Part model, mm, in its own coordinate system. A direction names the side the tool comes from. Give positions to 0.01 mm unless a question says otherwise; leave off trailing zeros. Loops run counter-clockwise (first coordinate to the right, second up) from the corner with the lowest first, then second, coordinate; pieces in that order, holes last. Notation, with made-up numbers: (26.25, -16) -> (31.25, -16) arc R25 cw to (31.25, -2) -> close; hole circle Ø9 at (8.25, 69). An arc over 180 degrees is marked (long way). Write item = value, one per line.
from build123d import *

# Parameters (mm, degrees)
BOSS_EXTRUDE1_DEPTH = 3
SKETCH2_R           = 16
BOSS_EXTRUDE2_DEPTH = 32
SKETCH3_R           = 13.8
BOSS_EXTRUDE3_DEPTH = 38
SKETCH4_R           = 18
SKETCH4_R_2         = 13.8
BOSS_EXTRUDE4_DEPTH = 17


with BuildPart() as part:
    # Sketch1 → Boss-Extrude1 (new body)
    with BuildSketch(Plane.XY):
        with BuildLine():
            Line((-4.002811512, 9), (4.002811512, 9))
            ThreePointArc((4.002811512, 9), (9.85, 0), (4.002811512, -9))
            Line((4.002811512, -9), (-4.002811512, -9))
            ThreePointArc((-4.002811512, -9), (-9.85, 0), (-4.002811512, 9))
        make_face()
    extrude(amount=BOSS_EXTRUDE1_DEPTH)

    # Sketch2 → Boss-Extrude2 (add)
    with BuildSketch(Plane(origin=(0, 0, 0), x_dir=(-1, 0, 0), z_dir=(0, 0, -1))):
        Circle(SKETCH2_R)
    extrude(amount=BOSS_EXTRUDE2_DEPTH)

    # Sketch3 → Boss-Extrude3 (add)
    with BuildSketch(Plane(origin=(0, 0, -32), x_dir=(-1, 0, 0), z_dir=(0, 0, -1))):
        Circle(SKETCH3_R)
    extrude(amount=BOSS_EXTRUDE3_DEPTH)

    # Sketch4 → Boss-Extrude4 (add)
    # profile 1 of 3: a face of its own
    with BuildSketch(Plane(origin=(0, 0, -70), x_dir=(-1, 0, 0), z_dir=(0, 0, -1))):
        Circle(SKETCH4_R)
        Circle(SKETCH4_R_2, mode=Mode.SUBTRACT)
    # profile 2 of 3: a face of its own
    with BuildSketch(Plane(origin=(0, 0, -70), x_dir=(-1, 0, 0), z_dir=(0, 0, -1))):
        Circle(SKETCH4_R_2)
    # profile 3 of 3: a face of its own
    with BuildSketch(Plane(origin=(0, 0, -70), x_dir=(-1, 0, 0), z_dir=(0, 0, -1))):
        with BuildLine():
            Line((-17.654073056, -3.511937432), (-30.0520382, -15.909902577))
            Line((-30.0520382, -15.909902577), (-15.909902577, -30.0520382))
            Line((-15.909902577, -30.0520382), (-3.511937432, -17.654073056))
            ThreePointArc((-3.511937432, -17.654073056), (-12.727922061, -12.727922061), (-17.654073056, -3.511937432))
        make_face()
    extrude(amount=BOSS_EXTRUDE4_DEPTH)


solid = part.part
1) Slice it at D-D, the plane x = -11. List the corners of the cut face in (y, z).
Resolved:
outline = (-14.25, -87) -> (14.25, -87) -> (14.25, -70) -> (8.33, -70) -> (8.33, -32) -> (11.62, -32) -> (11.62, 0) -> (-11.62, 0) -> (-11.62, -32) -> (-8.33, -32) -> (-8.33, -70) -> (-14.25, -70) -> close
2) Slice it at A-A, the plane y = 0. List the corners of the cut face in (x, z), and give its area (3 significant figures).
Resolved:
outline = (-18, -87) -> (18, -87) -> (18, -70) -> (13.8, -70) -> (13.8, -32) -> (16, -32) -> (16, 0) -> (9.85, 0) -> (9.85, 3) -> (-9.85, 3) -> (-9.85, 0) -> (-16, 0) -> (-16, -32) -> (-13.8, -32) -> (-13.8, -70) -> (-18, -70) -> close
area = 2,740 mm²
3) Drop flat-ended pins along their axis: P1, Ø1.5, axis at x = -6, z = -22, coming from the -Y side; P2, Ø3.5, axis at x = -1.5, z = 1.5, coming from the +Y side; P3, Ø1, axis at x = 12.5, z = -29, coming from the -Y side. Give the stop position or say it passes through.
Resolved:
P1 = -15.11
P2 = 15.99
P3 = -10.58
4) Drill centre lines: line 1 along X through (y, z) = (-0.5, -30.5); line 2 along Z through (x, y) = (-7, -9.5); line 3 along X through (y, z) = (-14.5, -80). Where is each one in solid material? Low to high. Write a range as [from, to].
Resolved:
line_1 = [-15.99, 15.99]
line_2 = [-87, 0]
line_3 = [-10.67, 28.64]
5) Slice it at B-B, the plane x = 0. List the corners of the cut face in (y, z), and give its area (3 significant figures).
Resolved:
outline = (-18, -87) -> (18, -87) -> (18, -70) -> (13.8, -70) -> (13.8, -32) -> (16, -32) -> (16, 0) -> (9, 0) -> (9, 3) -> (-9, 3) -> (-9, 0) -> (-16, 0) -> (-16, -32) -> (-13.8, -32) -> (-13.8, -70) -> (-18, -70) -> close
area = 2,740 mm²
6) Which spindle directions (+Z, -Z, +X, -X, +Y, -Y) get a long thin tool onto all of the face, cutting with end or side? Do faces 4 (the face through (3.47, -15.62, -15.78)), 5 (the face through (1.796, 13.683, -50.734)), 6 (the face through (9.85, 0.16, 1.48)), 7 (the face through (0, -9, 1)), 8 (the face through (0, 9, 1)). Say none if no direction does.
Resolved:
face_4 = +Z
face_5 = none
face_6 = +Z, +X
face_7 = +Z, +X, -X, -Y
face_8 = +Z, +X, -X, +Y
7) Slice it at C-C, the plane z = -25. List the corners of the cut face in (x, y), and give its area (3 significant figures).
Resolved:
outline = circle Ø32 at (0, 0)
area = 804 mm²
8) Pull direction Z, two halves, no side cores. Call faces 1 (the face through (8, -13, -70)), 2 (the face through (-6.9, 7.3, 0)), 3 (the face through (-9.85, -0.16, 1.48)): pulls with the +Z half, pulls with the -Z half, needs draft (parallel to the pull), parting line crosses it, or undercut.
Resolved:
face_1 = undercut
face_2 = pulls with the +Z half
face_3 = needs draft
